```python
from build123d import *

# Parameters (mm, degrees)
SKETCH1_R           = 28
BOSS_EXTRUDE1_DEPTH = 24
SKETCH6_R           = 1.9
CUT_EXTRUDE6_DEPTH  = 24
CUT_EXTRUDE7_DEPTH  = 24
CIRPATTERN1_COUNT   = 6
SKETCH17_R          = 1.5
CUT_EXTRUDE9_DEPTH  = 8
SKETCH18_R          = 1.607527434
CUT_EXTRUDE10_DEPTH = 8


with BuildPart() as part:
    # Sketch1 → Boss-Extrude1 (new body)
    with BuildSketch(Plane(origin=(0, 0, 0), x_dir=(1, 0, 0), z_dir=(0, 1, 0))):
        with Locations(Location((0, 0, 0), (0, 0, 270))):
            Circle(SKETCH1_R)
    extrude(amount=BOSS_EXTRUDE1_DEPTH)

    # Sketch6 → Cut-Extrude6 (cut)
    with BuildSketch(Plane(origin=(0, 0, 0), x_dir=(1, 0, 0), z_dir=(0, 1, 0))):
        with Locations(Location((0, 0, 0), (0, 0, 270))):
            Circle(SKETCH6_R)
    extrude(amount=CUT_EXTRUDE6_DEPTH, mode=Mode.SUBTRACT)

    # Sketch3 → Cut-Extrude7 (cut)
    with BuildSketch(Plane(origin=(0, 0, 0), x_dir=(1, 0, 0), z_dir=(0, 1, 0))):
        with BuildLine():
            Line((6.025985397, 9.5), (20.264254242, 9.5))
            ThreePointArc((20.264254242, 9.5), (21.992584206, 10.493582822), (22.003675207, 12.487124464))
            ThreePointArc((22.003675207, 12.487124464), (16.353652552, 19.304094079), (8.700746754, 23.756830721))
            ThreePointArc((8.700746754, 23.756830721), (7.330784322, 23.758890252), (6.280889879, 22.878820388))
            Line((6.280889879, 22.878820388), (1.119750126, 13.939464109))
            ThreePointArc((1.119750126, 13.939464109), (1.021677147, 12.132837227), (2.421340415, 10.986337451))
            ThreePointArc((2.421340415, 10.986337451), (4.288546152, 10.400522675), (6.025985397, 9.5))
        make_face()
    cut_extrude7 = extrude(amount=CUT_EXTRUDE7_DEPTH, mode=Mode.SUBTRACT)

    # CirPattern1: Cut-Extrude7 ×6 about axis
    cirpattern1_axis = Axis((0, 0, 0), (0, 1, 0))
    for i in range(1, CIRPATTERN1_COUNT):
        add(cut_extrude7.rotate(cirpattern1_axis, i * 360 / CIRPATTERN1_COUNT), mode=Mode.SUBTRACT)

    # Sketch14 → Revolve1 (revolve)
    with BuildSketch(Plane.XY):
        Polygon((25.5, 13), (25.5, 12), (28, 12), (28, 14), align=None)
    revolve1 = revolve(axis=Axis((0, 24, 0), (0, -1, 0)))

    # Mirror11: Revolve1 across plane
    add(revolve1.mirror(Plane.ZX.offset(12)))

    # Sketch15 → Cut-Revolve5 (revolve, cut)
    with BuildSketch(Plane.XY, mode=Mode.PRIVATE) as cut_revolve5_sk:
        Polygon((5, 8), (5, 0), (0, 0), (0, 8), (0, 24), (25, 24), (14, 8), align=None)
    revolve(cut_revolve5_sk.sketch.rotate(Axis((0, 8, 0), (0, -1, 0)), 90), axis=Axis((0, 8, 0), (0, -1, 0)), mode=Mode.SUBTRACT)

    # Sketch17 → Cut-Extrude9 (cut)
    with BuildSketch(Plane(origin=(0, 0, 0), x_dir=(1, 0, 0), z_dir=(0, 1, 0))):
        with Locations(Location((0, 8, 0), (0, 0, 270))):
            Circle(SKETCH17_R)
        with Locations(Location((8, 0, 0), (0, 0, 270))):
            Circle(SKETCH17_R)
        with Locations(Location((0, -8, 0), (0, 0, 270))):
            Circle(SKETCH17_R)
        with Locations(Location((-8, 0, 0), (0, 0, 270))):
            Circle(SKETCH17_R)
    extrude(amount=CUT_EXTRUDE9_DEPTH, mode=Mode.SUBTRACT)

    # Sketch18 → Cut-Extrude10 (cut)
    with BuildSketch(Plane(origin=(0, 0, 0), x_dir=(1, 0, 0), z_dir=(0, 1, 0))):
        with Locations((3.080772614, 3.800674665)):
            Circle(SKETCH18_R)
        with Locations((-3.080772614, -3.800674665)):
            Circle(SKETCH18_R)
    extrude(amount=CUT_EXTRUDE10_DEPTH, mode=Mode.SUBTRACT)


solid = part.part
```
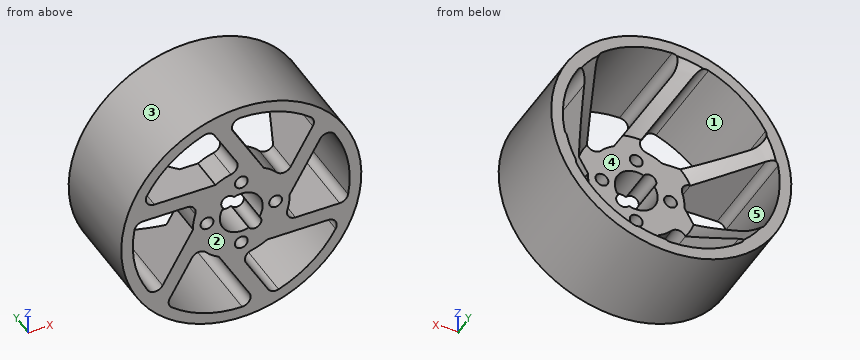
Here's how the part is built. I have some questions about the finished solid (model axes, mm). Face numbers are marked on the shaded views. A direction names the side the tool comes from. Give positions to 0.01 mm unless a question says otherwise; leave off trailing zeros. Use one line per item in the form item = value. Start each with the question number.
1) Imagine slicing it at A-A (y = 6). Count the separate pieces of the cut face and the enclosed holes in it, then the cut area to 3 significant figures.
2) Which directions (+Z, -Z, +X, -X, +Y, -Y) give clear straight access to the entire face, cutting with the end or side of a thin tool? Please do the marked faces 4 and 5.
3) For P1, Ø4, axis at y = 11, z = -16.5, coming from the -X side; P2, Ø5, axis at x = 3.08, z = -3.8, coming from the +Y side; P3, Ø6, axis at y = 9, z = 8.5, coming from the -X side, each with a flat end and sliding along its axis, tell me the tip position at first contact or that it passes through.
4) Thinking about a two-plate mould opening in Z: for the marked faces 1, 2 and 3, which applies, +Z half, -Z half, draft (parallel to the pull), parting line (faces both ways), or undercut?
5) Please list where these lines run through material, in increasing order: line 1 along X through (y, z) = (2.5, 0); line 2 along X through (y, z) = (16.25, 11.5); line 3 along X through (y, z) = (11.75, -7.5).
Check values:
q1.separate_pieces = 1
q1.enclosed_holes = 11
q1.area = 1,100 mm^2
q2.face_4 = +Y
q2.face_5 = +Y, -Y
q3.P1 = -23.95
q3.P2 = 8
q3.P3 = -27.45
q4.face_1 = undercut
q4.face_2 = draft
q4.face_3 = parting line
q5.line_1 = -28 to -25.3, -11.25 to -9.5, -6.5 to -5, 5 to 6.5, 9.5 to 11.25, 25.3 to 28
q5.line_2 = -25.53 to -22.26, 15.96 to 17.61, 22.54 to 25.53
q5.line_3 = -26.98 to -24.16, -15.3 to -14.78, 14.78 to 26.98
